Read the model definition and answer for the solid it produces. Units are mm, in the model's axes. A direction names the side the tool comes from. Give positions to 0.01 mm unless a question says otherwise; leave off trailing zeros. Loops run counter-clockwise (first coordinate to the right, second up) from the corner with the lowest first, then second, coordinate; pieces in that order, holes last. Notation, with made-up numbers: (53, 18) - (77, 18) arc R10 ccw to (77, 24) - close; hole circle Ø2 at (-35.5, -20). An arc over 180 degrees is marked (long way). Write each question's results on one line, items separated by ' | '. Start each with the question number.
Q1. Find the intervals of material crossed by line 1 (Y direction, x = 84, z = -25); line 2 (X direction, y = 8, z = -32); line 3 (X direction, y = 0, z = -2), in increasing order. Write a range as from..to.
Q2. Determine the mould class of faces 1 (the flat face through (27, -16, -34)), 2 (the cylindrical face through (41.41, 45.72, -4.51)), 3 (the flat face through (43, 50, -20)) for opening direction Z: +Z half, -Z half, draft (parallel to the pull), parting line (faces both ways), or undercut.
Q3. Given pin 1 (3 mm diameter, centred on x = 106.5, y = -32.5, fed in from +Z); pin 2 (8 mm diameter, centred on x = 4, z = -8.5, fed in from -Y); pin 3 (5 mm diameter, centred on y = -35.5, z = -27, fed in from -X); pin 4 (14 mm diameter, centred on x = 84, y = 0, fed in from +Z), each flat-ended and moving along its own axis, determine where each tip first touches the part or whether it passes through.
Q4. For faces 4 (the flat face through (41, -50, -20)), 5 (the conical face through (-35.055, -11.039, -20.366)), 6 (the cylindrical face through (98.307, -4.506, -30.14)), determine the directions among +Z, -Z, +X, -X, +Y, -Y from which every point of the face is accessible in a straight line to the end or side of a thin tool.
Q5. The part is cut by section C-C, the plane z = -8. Write down the section's boundary in (x, y).
Q6. The part is cut by section A-A, the plane x = 57.5. Write down the section's boundary in (y, z), plus the area to 3 significant figures.
Q7. The part is cut by section B-B, the plane y = 0. State how many separate pieces and enclosed holes the cut face has, plus the area to 3 significant figures.
```python
from build123d import *

# Parameters (mm, degrees)
F0_R           = 31
F0_R_2         = 8.75
F2_DEPTH       = 40
F4_D           = 17.5
F4_DEPTH       = 50
F4_CBORE_D     = 30
F4_CBORE_DEPTH = 20
F6_R           = 3
F8_R           = 15
F9_R           = 2


with BuildPart() as f2:
    # F0 (on Top) → F2 (new body)
    with BuildSketch(Plane.XY):
        with BuildLine():
            Line((84, 50), (0, 50))
            ThreePointArc((0, 50), (-50, 0), (0, -50))
            Line((0, -50), (84, -50))
            ThreePointArc((84, -50), (134, 0), (84, 50))
        make_face()
        Circle(F0_R, mode=Mode.SUBTRACT)
        with Locations((84, 0)):
            Circle(F0_R_2, mode=Mode.SUBTRACT)
    extrude(amount=-F2_DEPTH)

    # F4
    with Locations(Plane(origin=(0, 0, -40), x_dir=(1, 0, 0), z_dir=(0, 0, -1))):
        with Locations((84, 0)):
            CounterBoreHole(F4_D / 2, F4_CBORE_D / 2, F4_CBORE_DEPTH, depth=F4_DEPTH)


with BuildPart() as f5:
    # F1 (on Front) → F5 (revolve)
    with BuildSketch(Plane.XZ):
        Polygon((0, 0), (-31, 0), (-31, -6), (-36.600505, -6), (-39.5, -13), (-36.600505, -20), (-39.5, -27), (-36.58464, -33.999979), (-31, -33.999979), (-31, -40), (0, -40), align=None)
    revolve(axis=Axis((0, 0, -20), (0, 0, 1)))

    # F6
    f6_edges = [f5.edges().sort_by_distance(p)[0] for p in [
        (39.5, 0, -27),
        (39.5, 0, -13),
    ]]
    fillet(f6_edges, radius=F6_R)


with BuildPart() as f2_1:
    add(f2.part)

    # F7: cut F5
    add(f5.part, mode=Mode.SUBTRACT)

    # F8
    f8_edges = [f2_1.edges().sort_by_distance(p)[0] for p in [
        (42, -50, 0),
        (42, -50, -40),
    ]]
    fillet(f8_edges, radius=F8_R)

    # F9
    f9_edges = [f2_1.edges().sort_by_distance(p)[0] for p in [
        (-31, 0, 0),
    ]]
    fillet(f9_edges, radius=F9_R)


solid = f2_1.part
```
Check sheet entries:
1) line 1: y = -50..-15, 15..50 | line 2: x = -47.6..-36.55, 36.55..71.31, 96.69..131.6 | line 3: x = -42.48..-31, 31..75.25, 92.75..126.48
2) face 1: undercut | face 2: +Z half | face 3: draft
3) pin 1: stops at z = -0.31 | pin 2: stops at y = -49.79 | pin 3: stops at x = -37.42 | pin 4: passes through
4) face 4: +Z, -Z, +X, -X, -Y | face 5: none | face 6: -Z
5) outline: (0, -48.27) - (84, -48.27) arc R48.27 ccw to (84, 48.27) - (0, 48.27) arc R48.27 ccw to start; hole circle Ø74.86 at (0, 0); hole circle Ø17.5 at (84, 0)
6) outline: (-50, -25) arc R15 ccw to (-35, -40) - (35, -40) arc R15 ccw to (50, -25) - (50, -15) arc R15 ccw to (35, 0) - (-35, 0) arc R15 ccw to (-50, -15) - close | area: 3,810 mm^2
7) separate pieces: 3 | enclosed holes: 0 | area: 3,340 mm^2
